Here's the drawing with two shaded views (mm, measured from the low corner). I have some questions. Give positions to 0.01 mm unless a question says otherwise; leave off trailing zeros. Loops run counter-clockwise (first coordinate to the right, second up) from the corner with the lowest first, then second, coordinate; pieces in that order, holes last. Notation, with made-up numbers: M 60,18.5 L 64,18.5 A21 ccw 64,45.5 Z; hole C 62.5,-13 d2. An arc over 180 degrees is marked long. Use CSV: the item, a comma, the result in double quotes.
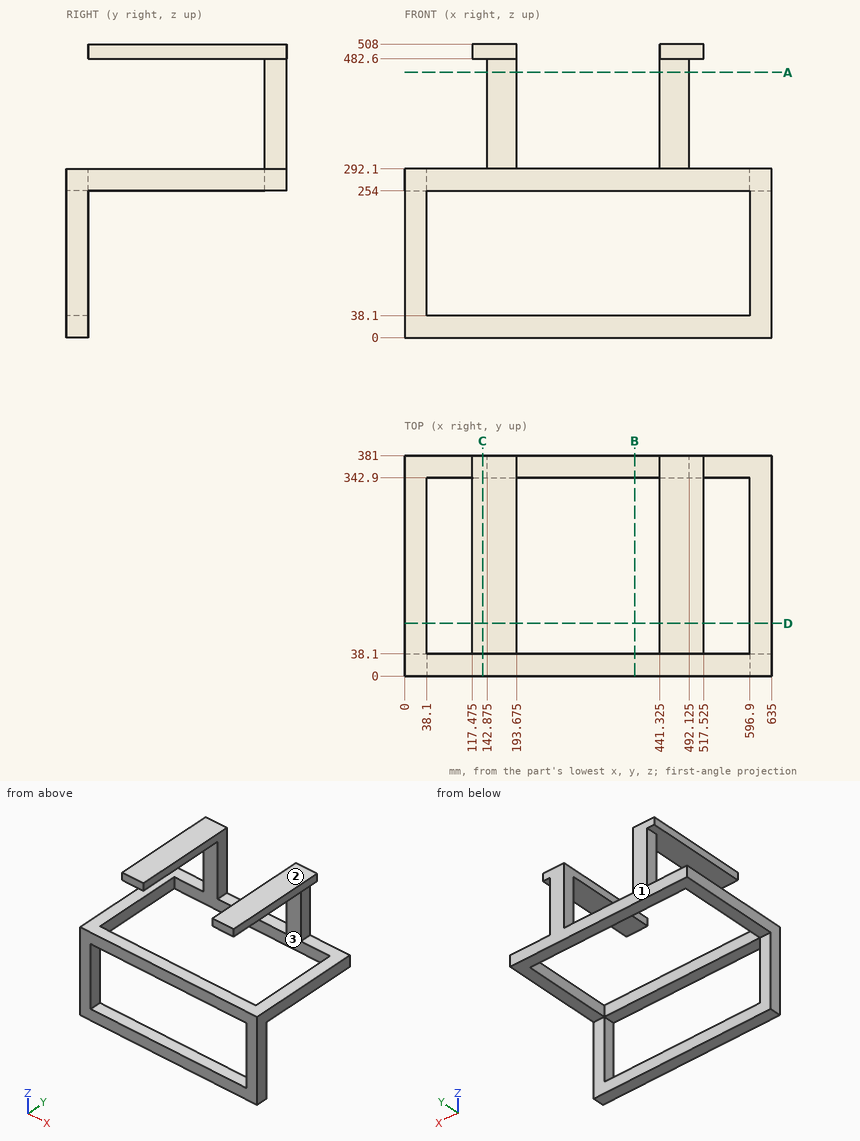
1. I want a section at B-B, the plane x = 398. List the corners of the cut face in (y, z) for me.
Outcome:
outline,"M 0,0 L 38.1,0 L 38.1,38.1 L 0,38.1 Z; M 0,254 L 38.1,254 L 38.1,292.1 L 0,292.1 Z; M 342.9,254 L 381,254 L 381,292.1 L 342.9,292.1 Z"
2. I want a section at A-A, the plane z = 459. List the corners of the cut face in (x, y) for me (3 decimals), then the cut area to 3 significant figures.
Outcome:
outline,"M 142.875,342.9 L 193.675,342.9 L 193.675,381 L 142.875,381 Z; M 441.325,342.9 L 492.125,342.9 L 492.125,381 L 441.325,381 Z"
area,"3,870 mm2"
3. I want a section at D-D, the plane y = 91. List the corners of the cut face in (x, z) for me (3 decimals).
Outcome:
outline,"M 0,254 L 38.1,254 L 38.1,292.1 L 0,292.1 Z; M 117.475,482.6 L 193.675,482.6 L 193.675,508 L 117.475,508 Z; M 441.325,482.6 L 517.525,482.6 L 517.525,508 L 441.325,508 Z; M 596.9,254 L 635,254 L 635,292.1 L 596.9,292.1 Z"
4. I want a section at C-C, the plane x = 135. List the corners of the cut face in (y, z) for me.
Outcome:
outline,"M 0,0 L 38.1,0 L 38.1,38.1 L 0,38.1 Z; M 0,254 L 38.1,254 L 38.1,292.1 L 0,292.1 Z; M 38.1,482.6 L 381,482.6 L 381,508 L 38.1,508 Z; M 342.9,254 L 381,254 L 381,292.1 L 342.9,292.1 Z"
5. I'm going to push flat-ended pins straight in: pin 1 Ø8 at (x, y) = (132.5, 334) entering from -Z; pin 2 Ø11.5 at (x, y) = (268.5, 21.5) entering from +Z; pin 3 Ø6 at (x, z) = (543, 254) entering from -Y; pin 4 Ø7.5 at (x, z) = (475, 496) entering from -Y. Where does each tip first touch, or does it pass through?
Outcome:
pin 1,"z = 482.6"
pin 2,"z = 292.1"
pin 3,"y = 0"
pin 4,"y = 38.1"
6. Please list where these lines run through material, in increasing order: line 1 (X direction, y = 233, z = 263.5); line 2 (Y direction, x = 567, z = 268); line 3 (Y direction, x = 457, z = 33).
Outcome:
line 1,"0 to 38.1, 596.9 to 635"
line 2,"0 to 38.1, 342.9 to 381"
line 3,"0 to 38.1"
7. If we mould it in two halves opening along Y, with no side actions, what happens to the marked faces 1, 2 and 3? For each: +Y half, -Y half, draft (parallel to the pull), parting line (faces both ways), or undercut.
Outcome:
face 1,"+Y half"
face 2,"draft"
face 3,"undercut"
